Here's the drawing with two shaded views (mm, measured from the low corner). I have some questions. A direction names the side the tool comes from. Give positions to 0.01 mm unless a question says otherwise; leave off trailing zeros. Write each loop counter-clockwise with the first axis right and the second up, starting at its lowest first coordinate (ties: lowest second). Pieces come first, ordered by that corner, then holes.
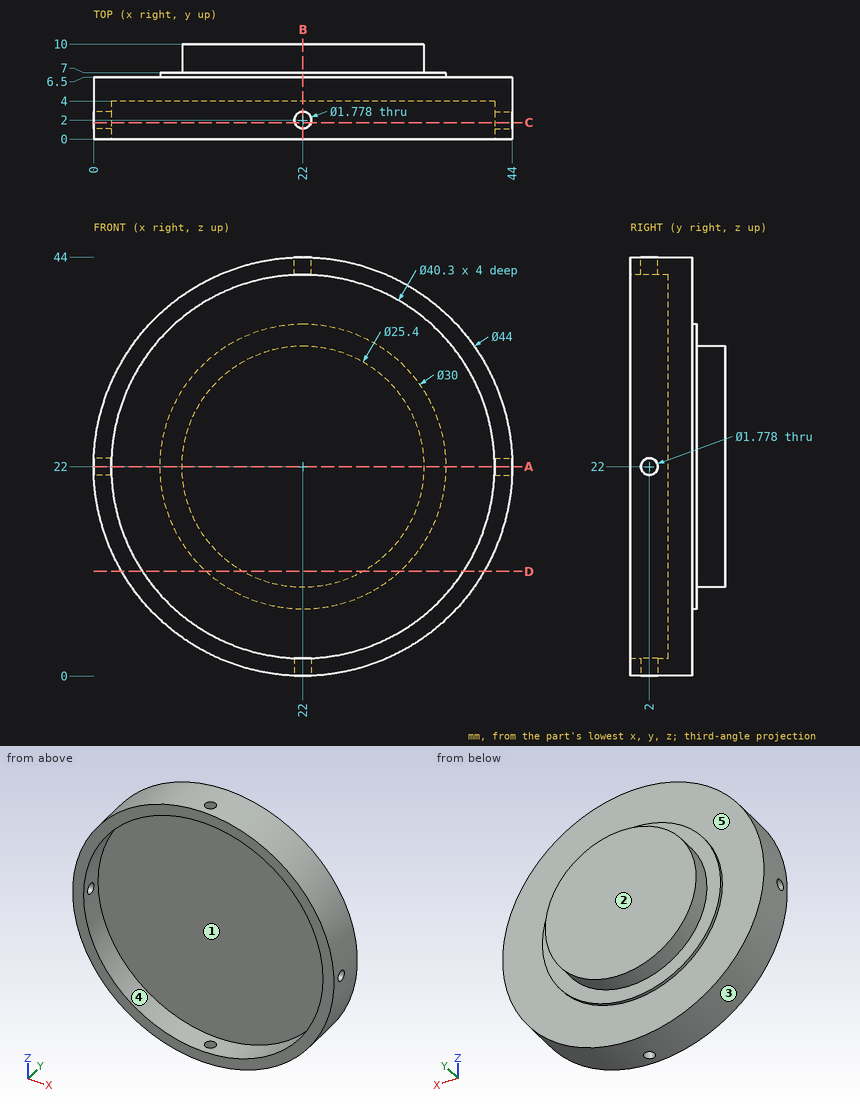
(1) Imagine slicing it at D-D, the plane z = 11. Write out the boundary of the cut face in (x, y).
Returned:
outline: (2.95, 0) - (5.12, 0) - (5.12, 4) - (38.88, 4) - (38.88, 0) - (41.05, 0) - (41.05, 6.5) - (32.2, 6.5) - (32.2, 7) - (28.35, 7) - (28.35, 10) - (15.65, 10) - (15.65, 7) - (11.8, 7) - (11.8, 6.5) - (2.95, 6.5) - close
(2) If we mould it in two halves opening along Z, with no side actions, what happens to the marked faces 3, 4 and 5? For each: +Z half, -Z half, draft (parallel to the pull), parting line (faces both ways), or undercut.
Returned:
face 3: parting line
face 4: undercut
face 5: draft
(3) Imagine slicing it at B-B, the plane x = 22. Write out the boundary of the cut face in (y, z), plus the area to 3 significant figures.
Returned:
outline: (0, 0) - (1.11, 0) - (1.11, 1.85) - (0, 1.85) - close; (0, 42.15) - (1.11, 42.15) - (1.11, 44) - (0, 44) - close; (2.89, 0) - (6.5, 0) - (6.5, 7) - (7, 7) - (7, 9.3) - (10, 9.3) - (10, 34.7) - (7, 34.7) - (7, 37) - (6.5, 37) - (6.5, 44) - (2.89, 44) - (2.89, 42.15) - (4, 42.15) - (4, 1.85) - (2.89, 1.85) - close
area: 209 mm2
(4) Will these pins go through, and if not, where does the flat tip stop? P1, Ø6, axis at x = 31.5, z = 33.5, coming from the -Y side; P2, Ø2, axis at x = 14.5, y = 4.5, coming from the -Z side; P3, Ø3, axis at y = 6.5, z = 7, coming from the -X side.
Returned:
P1: stops at y = 4
P2: stops at z = 0.98
P3: stops at x = 4.63
(5) If I drill on L1, parallel to Z at x = 22.5, y = 3.25; L2, parallel to Y at x = 28.5, z = 37; L3, parallel to Y at x = 13, z = 31, over which ranges is the centre line in solid material (lowest first)?
Returned:
L1: z = 0.01 to 1.86, 42.14 to 43.99
L2: y = 4 to 6.5
L3: y = 4 to 7
(6) For the marked faces 1 and 2, which set-ups out of +Z, -Z, +X, -X, +Y, -Y let a thin tool reach every point of the face, with its end or its side?
Returned:
face 1: -Y
face 2: +Z, -Z, +X, -X, +Y
(7) Imagine slicing it at A-A, the plane z = 22. Write out the boundary of the cut face in (x, y).
Returned:
outline: (0, 0) - (1.85, 0) - (1.85, 1.11) - (0, 1.11) - close; (0, 2.89) - (1.85, 2.89) - (1.85, 4) - (42.15, 4) - (42.15, 2.89) - (44, 2.89) - (44, 6.5) - (37, 6.5) - (37, 7) - (34.7, 7) - (34.7, 10) - (9.3, 10) - (9.3, 7) - (7, 7) - (7, 6.5) - (0, 6.5) - close; (42.15, 0) - (44, 0) - (44, 1.11) - (42.15, 1.11) - close
(8) Imagine slicing it at C-C, the plane y = 1.75. Write out the boundary of the cut face in (x, z), plus the area to 3 significant figures.
Returned:
outline: (0.02, 21.15) arc R22 ccw to (21.15, 0.02) - (21.15, 1.87) arc R20.15 cw to (1.87, 21.15) - close; (0.02, 22.85) - (1.87, 22.85) arc R20.15 cw to (21.15, 42.13) - (21.15, 43.98) arc R22 ccw to start; (22.85, 0.02) arc R22 ccw to (43.98, 21.15) - (42.13, 21.15) arc R20.15 cw to (22.85, 1.87) - close; (22.85, 42.13) arc R20.15 cw to (42.13, 22.85) - (43.98, 22.85) arc R22 ccw to (22.85, 43.98) - close
area: 232 mm2
